For this review, take the finished solid that the model builds, in its own axes (mm). A direction names the side the tool comes from. Round coordinates to 2 decimals unless told otherwise and drop trailing zeros. Order: outer loops, then holes, each group sorted by start corner. A loop starts at its lowest first (then second) coordinate and runs counter-clockwise, first axis right, second up. Notation, with made-up numbers: (-16, -18) -> (19, -18) arc R14 cw to (19, -7) -> close; hole circle Ø8 at (-15.5, 61). An arc over 180 degrees is marked (long way). Put each result on its own line as item: value. Start each with the question number.
```python
from build123d import *

# Parameters (mm, degrees)
F1_DEPTH = 600
F2_R     = 100
F3_DEPTH = 500


with BuildPart() as f1:
    # F0 (on Right) → F1 (new body)
    with BuildSketch(Plane.YZ):
        with BuildLine():
            Line((250, 0), (175.481897, 330.558985))
            ThreePointArc((175.481897, 330.558985), (0, 470.885545), (-175.481897, 330.558985))
            Line((-175.481897, 330.558985), (-250, 0))
            Line((-250, 0), (250, 0))
        make_face()
    extrude(amount=F1_DEPTH)

    # F2 (on face) → F3 (cut)
    with BuildSketch(Plane.YZ.offset(600)):
        with Locations((0, 291)):
            Circle(F2_R)
    extrude(amount=-F3_DEPTH, mode=Mode.SUBTRACT)


solid = f1.part
```
Item 1: Consider section A-A, the plane x = 424. Write out the cut boundary in (y, z), plus the area to 3 significant figures.
Item 2: Mouldability with a two-part tool opening along Z and no side actions: class faces 3 (the face through (296, -3, 0)), 4 (the face through (100, -1, 292)), 5 (the face through (295.8, -212.22, 167.59)) as +Z half, -Z half, draft (parallel to the pull), parting line (faces both ways), or undercut.
Item 3: Consider section B-B, the plane y = 0. Write out the cut boundary in (x, z).
Item 4: Consider section D-D, the plane y = -133. Write out the cut boundary in (x, z), plus the area to 3 significant figures.
Item 5: Consider section C-C, the plane z = 291. Write out the cut boundary in (x, y), plus the area to 3 significant figures.
Item 6: Tool access review of faces 1 (the face through (353.5, -21.68, 193.38)), 2 (the face through (295.8, 3.397, 470.853)): name each direction out of +Z, -Z, +X, -X, +Y, -Y from which nothing blocks a thin tool from reaching the whole face with its end or side.
Item 7: Insertion check: pin 1 Ø2 at (x, z) = (93.5, 342) entering from +Y; pin 2 Ø12 at (x, z) = (89.5, 325.5) entering from +Y; pin 3 Ø1.5 at (x, z) = (181.5, 166) entering from -Y; pin 4 Ø12 at (y, z) = (43, 270) entering from -X. Each pin has a flat end and moves straight along its axis. Give the tip position at first contact, or say it passes through.
Item 8: For L1, parallel to Y at x = 326, z = 254; L2, parallel to X at y = -90, z = 271; L3, parallel to Y at x = 448.5, z = 297, list the stretches that pass through material, from the lowest coordinate up.
Evaluation:
1. outline: (-250, 0) -> (250, 0) -> (175.48, 330.56) arc R179.89 ccw to (-175.48, 330.56) -> close; hole circle Ø200 at (0, 291)
1. area: 146,000 mm^2
2. face 3: -Z half
2. face 4: undercut
2. face 5: +Z half
3. outline: (0, 0) -> (600, 0) -> (600, 191) -> (100, 191) -> (100, 391) -> (600, 391) -> (600, 470.89) -> (0, 470.89) -> close
4. outline: (0, 0) -> (600, 0) -> (600, 412.12) -> (0, 412.12) -> close
4. area: 247,000 mm^2
5. outline: (0, -184.4) -> (600, -184.4) -> (600, -100) -> (100, -100) -> (100, 100) -> (600, 100) -> (600, 184.4) -> (0, 184.4) -> close
5. area: 121,000 mm^2
6. face 1: +X
6. face 2: +Z, +X, -X
7. pin 1: stops at y = 172.8
7. pin 2: stops at y = 177.97
7. pin 3: stops at y = -212.75
7. pin 4: stops at x = 0
8. L1: y = -192.74 to -92.9, 92.9 to 192.74
8. L2: x = 0 to 100
8. L3: y = -183.05 to -99.82, 99.82 to 183.05
